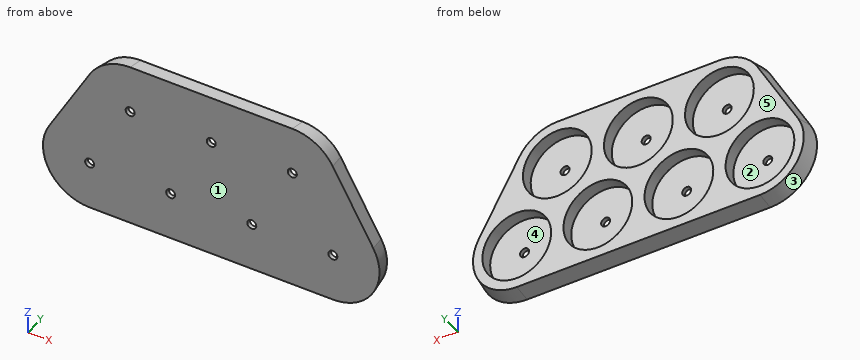
from build123d import *

# Parameters (mm, degrees)
BOSS_EXTRUDE1_DEPTH = 4
BOSS_EXTRUDE1_DRAFT = 10
CUT_EXTRUDE1_START  = 4
SKETCH1_3_R         = 1.1
CUT_EXTRUDE1_DEPTH  = 4
CUT_EXTRUDE2_START  = 4
SKETCH1_4_R         = 8.4
SKETCH1_4_R_2       = 1.1
CUT_EXTRUDE2_DEPTH  = 3


# Read off the part's stored shape, not the designer's step: Boss-Extrude1
with BuildPart() as part:
    # Boss-Extrude1 outline → Boss-Extrude1 (with draft: the straight prism first)
    with BuildSketch(Plane(origin=(0, 4, 0), x_dir=(1, 0, 0), z_dir=(0, 1, 0))):
        with BuildLine():
            ThreePointArc((-58.761875024, -22.494649034), (-54.847346039, -26.409178019), (-49.5, -27.841995072))
            Line((-49.5, -27.841995072), (-9.9, -27.841995072))
            ThreePointArc((-9.9, -27.841995072), (-4.552653961, -26.409178019), (-0.638124976, -22.494649034))
            Line((-0.638124976, -22.494649034), (9.261875024, -5.347346039))
            ThreePointArc((9.261875024, -5.347346039), (9.261875024, 5.347346039), (0, 10.694692077))
            Line((0, 10.694692077), (-59.4, 10.694692077))
            ThreePointArc((-59.4, 10.694692077), (-68.661875024, 5.347346039), (-68.661875024, -5.347346039))
            Line((-68.661875024, -5.347346039), (-58.761875024, -22.494649034))
        make_face()
    extrude(amount=-BOSS_EXTRUDE1_DEPTH)
    # Boss-Extrude1: the draft: its side faces are tilted about the plane it starts from
    boss_extrude1_sides = [part.faces().sort_by_distance(p)[0] for p in [
        (-68.661875024, 2, -5.347346038),
        (-63.711875024, 2, 13.920997536),
        (-54.847346038, 2, 26.409178019),
        (-29.7, 2, 27.841995072),
        (-4.552653962, 2, 26.409178019),
        (4.311875024, 2, 13.920997536),
        (9.261875024, 2, -5.347346038),
        (-29.7, 2, -10.694692077),
    ]]
    draft(boss_extrude1_sides, Plane(origin=(0, 4, 0), x_dir=(1, 0, 0), z_dir=(0, 1, 0)), BOSS_EXTRUDE1_DRAFT)

    # Sketch1<3> → Cut-Extrude1 (cut)
    with BuildSketch(Plane(origin=(0, 0, 0), x_dir=(1, 0, 0), z_dir=(0, 1, 0)).offset(CUT_EXTRUDE1_START)):
        with Locations(Location((-9.9, -17.147302995, 0), (0, 0, 270))):
            Circle(SKETCH1_3_R)
        with Locations(Location((0, 0, 0), (0, 0, 270))):
            Circle(SKETCH1_3_R)
        with Locations(Location((-29.7, -17.147302995, 0), (0, 0, 270))):
            Circle(SKETCH1_3_R)
        with Locations(Location((-39.6, 0, 0), (0, 0, 270))):
            Circle(SKETCH1_3_R)
        with Locations(Location((-49.5, -17.147302995, 0), (0, 0, 270))):
            Circle(SKETCH1_3_R)
        with Locations(Location((-59.4, 0, 0), (0, 0, 270))):
            Circle(SKETCH1_3_R)
        with Locations(Location((-19.8, 0, 0), (0, 0, 270))):
            Circle(SKETCH1_3_R)
    extrude(amount=-CUT_EXTRUDE1_DEPTH, mode=Mode.SUBTRACT)

    # Sketch1<4> → Cut-Extrude2 (cut)
    # profile 1 of 7: a face of its own
    with BuildSketch(Plane(origin=(0, 0, 0), x_dir=(1, 0, 0), z_dir=(0, 1, 0)).offset(CUT_EXTRUDE2_START)):
        with Locations(Location((-19.8, 0, 0), (0, 0, 270))):
            Circle(SKETCH1_4_R)
        with Locations(Location((-19.8, 0, 0), (0, 0, 270))):
            Circle(SKETCH1_4_R_2, mode=Mode.SUBTRACT)
    # profile 2 of 7: a face of its own
    with BuildSketch(Plane(origin=(0, 0, 0), x_dir=(1, 0, 0), z_dir=(0, 1, 0)).offset(CUT_EXTRUDE2_START)):
        with Locations(Location((-9.9, -17.147302995, 0), (0, 0, 270))):
            Circle(SKETCH1_4_R)
        with Locations(Location((-9.9, -17.147302995, 0), (0, 0, 270))):
            Circle(SKETCH1_4_R_2, mode=Mode.SUBTRACT)
    # profile 3 of 7: a face of its own
    with BuildSketch(Plane(origin=(0, 0, 0), x_dir=(1, 0, 0), z_dir=(0, 1, 0)).offset(CUT_EXTRUDE2_START)):
        with Locations(Location((0, 0, 0), (0, 0, 270))):
            Circle(SKETCH1_4_R)
        with Locations(Location((0, 0, 0), (0, 0, 270))):
            Circle(SKETCH1_4_R_2, mode=Mode.SUBTRACT)
    # profile 4 of 7: a face of its own
    with BuildSketch(Plane(origin=(0, 0, 0), x_dir=(1, 0, 0), z_dir=(0, 1, 0)).offset(CUT_EXTRUDE2_START)):
        with Locations(Location((-29.7, -17.147302995, 0), (0, 0, 270))):
            Circle(SKETCH1_4_R)
        with Locations(Location((-29.7, -17.147302995, 0), (0, 0, 270))):
            Circle(SKETCH1_4_R_2, mode=Mode.SUBTRACT)
    # profile 5 of 7: a face of its own
    with BuildSketch(Plane(origin=(0, 0, 0), x_dir=(1, 0, 0), z_dir=(0, 1, 0)).offset(CUT_EXTRUDE2_START)):
        with Locations(Location((-39.6, 0, 0), (0, 0, 270))):
            Circle(SKETCH1_4_R)
        with Locations(Location((-39.6, 0, 0), (0, 0, 270))):
            Circle(SKETCH1_4_R_2, mode=Mode.SUBTRACT)
    # profile 6 of 7: a face of its own
    with BuildSketch(Plane(origin=(0, 0, 0), x_dir=(1, 0, 0), z_dir=(0, 1, 0)).offset(CUT_EXTRUDE2_START)):
        with Locations(Location((-49.5, -17.147302995, 0), (0, 0, 270))):
            Circle(SKETCH1_4_R)
        with Locations(Location((-49.5, -17.147302995, 0), (0, 0, 270))):
            Circle(SKETCH1_4_R_2, mode=Mode.SUBTRACT)
    # profile 7 of 7: a face of its own
    with BuildSketch(Plane(origin=(0, 0, 0), x_dir=(1, 0, 0), z_dir=(0, 1, 0)).offset(CUT_EXTRUDE2_START)):
        with Locations(Location((-59.4, 0, 0), (0, 0, 270))):
            Circle(SKETCH1_4_R)
        with Locations(Location((-59.4, 0, 0), (0, 0, 270))):
            Circle(SKETCH1_4_R_2, mode=Mode.SUBTRACT)
    extrude(amount=-CUT_EXTRUDE2_DEPTH, mode=Mode.SUBTRACT)


solid = part.part
Geometry: final body of the model. Coordinates: model frame, mm. Face numbers are marked on the shaded views. A direction names the side the tool comes from. Coordinates: 2 decimals unless noted, no trailing zeros. Order: outer loops, then holes, each group sorted by start corner. A loop starts at its lowest first (then second) coordinate and runs counter-clockwise, first axis right, second up.
(1) Section query D-D (z = 21). Return the cut outline in (x, y), plus the area to 3 significant figures.
(2) Section query C-C (z = 0). State how many separate pieces and enclosed holes the cut face has, plus the area to 3 significant figures.
(3) Draft query along X for the marked faces 3, 4 and 5. Return one class per face: pulls with the +X half, pulls with the -X half, needs draft (parallel to the pull), parting line crosses it, or undercut.
(4) Section query A-A (x = -29.7). Return the cut outline in (y, z).
(5) Section query B-B (y = 1.8). Return the cut outline in (x, z).
(6) Material intervals for probe 1 along X at (y, z) = (2.2, 19); probe 2 along Z at (x, y) = (-27.5, 2.85); probe 3 along X at (y, z) = (0.45, 0), sorted ascending.
(7) Access query for the marked faces 1 and 2. Directions: +Z, -Z, +X, -X, +Y, -Y. A direction counts if a zero-diameter tool reaches every point of the face in a straight line with its end or side. Return the directions, or none.
(8) First-contact query: pin 1 (1.5 mm diameter, centred on x = -18, y = 1, fed in from +Z); pin 2 (8.5 mm diameter, centred on x = -31.5, z = 15.5, fed in from +Y); pin 3 (2 mm diameter, centred on x = -49.5, z = 17.15, fed in from +Y); pin 4 (1.5 mm diameter, centred on x = -36.5, y = 2, fed in from +Z). Flat tips, straight axial feed; report the tip coordinate or a pass-through.
Solution:
1. outline: (-60.44, 0) - (1.04, 0) - (0.22, 4) - (-2.44, 4) - (-2.44, 1) - (-17.36, 1) - (-17.36, 4) - (-22.24, 4) - (-22.24, 1) - (-37.16, 1) - (-37.16, 4) - (-42.04, 4) - (-42.04, 1) - (-56.96, 1) - (-56.96, 4) - (-59.62, 4) - close
1. area: 108 mm2
2. separate pieces: 5
2. enclosed holes: 0
2. area: 116 mm2
3. face 3: pulls with the -X half
3. face 4: undercut
3. face 5: needs draft
4. outline: (0, -11.4) - (4, -10.69) - (4, 8.75) - (1, 8.75) - (1, 16.05) - (0, 16.05) - close; (0, 18.25) - (1, 18.25) - (1, 25.55) - (4, 25.55) - (4, 27.84) - (0, 28.55) - close
5. outline: (-69, 5.54) arc R11.08 ccw to (-59.4, -11.08) - (0, -11.08) arc R11.08 ccw to (9.6, 5.54) - (-0.3, 22.69) arc R11.08 ccw to (-9.9, 28.23) - (-49.5, 28.23) arc R11.08 ccw to (-59.1, 22.69) - close; hole circle Ø16.8 at (-59.4, 0); hole circle Ø16.8 at (-49.5, 17.15); hole circle Ø16.8 at (-39.6, 0); hole circle Ø16.8 at (-29.7, 17.15); hole circle Ø16.8 at (-19.8, 0); hole circle Ø16.8 at (-9.9, 17.15); hole circle Ø16.8 at (0, 0)
6. probe 1: x = -61.15 to -57.69, -41.31 to -37.89, -21.51 to -18.09, -1.71 to 1.75
6. probe 2: z = -10.9 to -3.36, 3.36 to 9.04, 25.25 to 28.04
6. probe 3: x = -70.72 to -60.5, -58.3 to -40.7, -38.5 to -20.9, -18.7 to -1.1, 1.1 to 11.32
7. face 1: +Z, -Z, +X, -X, -Y
7. face 2: +Y
8. pin 1: stops at z = 28.5
8. pin 2: stops at y = 1
8. pin 3: passes through
8. pin 4: stops at z = 28.33
